Input: dimensioned drawing with shaded views. Units: mm. Origin: part minimum x, y, z. Give positions to 0.01 mm unless a question says otherwise; leave off trailing zeros. Order: outer loops, then holes, each group sorted by start corner. A loop starts at its lowest first (then second) coordinate and runs counter-clockwise, first axis right, second up. Notation, with made-up numbers: (67.5, 72) -> (82.5, 72) arc R14 ccw to (82.5, 91) -> close; hole circle Ø10 at (12, 31.5). An arc over 180 degrees is marked (long way). Use CSV: the item, a comma, the result in double quotes.
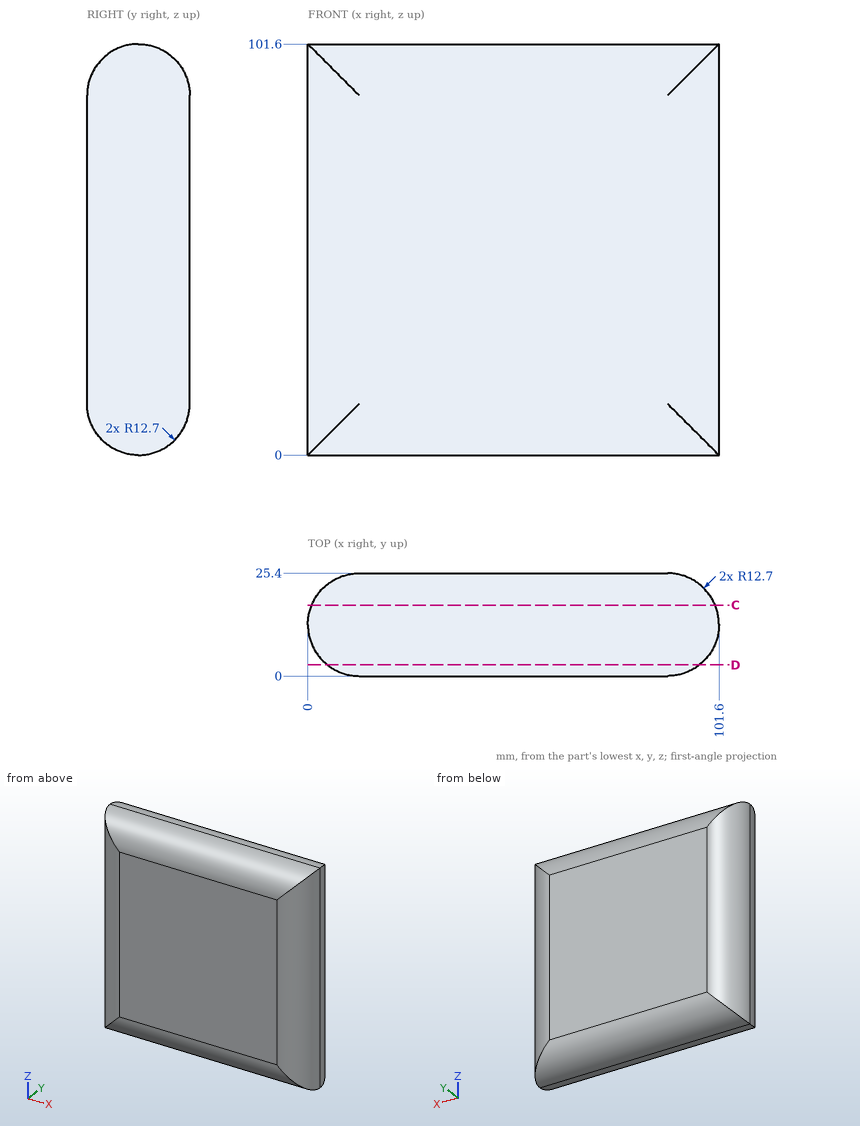
1. Pin query (flat end, axial travel): P1, Ø5, axis at x = 21, y = 4.5, coming from the -Z side; P2, Ø1.5, axis at y = 4.5, z = 35, coming from the -X side; P3, Ø6, axis at y = 8, z = 76.5, coming from the +X side. Return the tip coordinate at first contact, or that it passes through.
Answer below:
P1,"stops at z = 1.35"
P2,"stops at x = 2.41"
P3,"stops at x = 101.49"
2. Section query D-D on y = 2.75. Return loops of the section in (x, z).
Answer below:
outline,"(4.81, 4.81) -> (96.79, 4.81) -> (96.79, 96.79) -> (4.81, 96.79) -> close"
3. Ray query, line 1 along Y through (x, z) = (94, 38); line 2 along X through (y, z) = (14, 52.5); line 3 along X through (y, z) = (17.25, 21). Return the intervals inside material, ascending.
Answer below:
line 1,"y = 1.07 to 24.33"
line 2,"x = 0.07 to 101.53"
line 3,"x = 0.84 to 100.76"
4. Section query C-C on y = 17.5. Return loops of the section in (x, z), plus the area to 3 significant figures.
Answer below:
outline,"(0.94, 0.94) -> (100.66, 0.94) -> (100.66, 100.66) -> (0.94, 100.66) -> close"
area,"9,940 mm²"
